For this review, take the finished solid that the model builds, in its own axes (mm). A direction names the side the tool comes from. Round coordinates to 2 decimals unless told otherwise and drop trailing zeros. Order: outer loops, then holes, each group sorted by start corner. A loop starts at its lowest first (then second) coordinate and runs counter-clockwise, first axis right, second up. Notation, with made-up numbers: (-23, 77) -> (32, 77) arc R20 cw to (32, 85) -> close; hole circle Ø6 at (48.5, 15). An arc over 180 degrees is marked (long way). Answer in a Markdown table with one row per item.
```python
from build123d import *

# Parameters (mm, degrees)
SKETCH1_R           = 1.5
BOSS_EXTRUDE1_DEPTH = 4


with BuildPart() as part:
    # Sketch1 → Boss-Extrude1 (new body)
    with BuildSketch(Plane.XY):
        with BuildLine():
            Line((3.999999567, 13.999999851), (-4.33e-07, 13.999999851))
            Line((-4.33e-07, 13.999999851), (-4.33e-07, 4.999999851))
            Line((-4.33e-07, 4.999999851), (3.999999567, 4.999999851))
            Line((3.999999567, 4.999999851), (3.999999567, -1.49e-07))
            Line((3.999999567, -1.49e-07), (51.999999567, -1.49e-07))
            Line((51.999999567, -1.49e-07), (51.999999567, 4.999999851))
            Line((51.999999567, 4.999999851), (55.999999567, 4.999999851))
            Line((55.999999567, 4.999999851), (55.999999567, 13.999999851))
            Line((55.999999567, 13.999999851), (51.999999567, 13.999999851))
            Line((51.999999567, 13.999999851), (51.999999567, 18.999999851))
            ThreePointArc((51.999999567, 18.999999851), (49.656853817, 24.6568541), (43.999999567, 26.999999851))
            Line((43.999999567, 26.999999851), (11.999999567, 26.999999851))
            ThreePointArc((11.999999567, 26.999999851), (6.343145318, 24.6568541), (3.999999567, 18.999999851))
            Line((3.999999567, 18.999999851), (3.999999567, 13.999999851))
        make_face()
        with Locations((46.999999567, 18.299999851)):
            Circle(SKETCH1_R, mode=Mode.SUBTRACT)
        with Locations((46.999999567, 8.299999851)):
            Circle(SKETCH1_R, mode=Mode.SUBTRACT)
        with Locations((18.499999567, 18.299999851)):
            Circle(SKETCH1_R, mode=Mode.SUBTRACT)
        with Locations((18.499999567, 8.299999851)):
            Circle(SKETCH1_R, mode=Mode.SUBTRACT)
    extrude(amount=BOSS_EXTRUDE1_DEPTH)


solid = part.part
```
Q1. The part is to be moulded in two halves that separate along Y. For faces 4 (the face through (4, 17, 2)), 5 (the face through (17.3, 7.4, 2)), 6 (the face through (45.8, 7.4, 2)), 7 (the face through (49.719, 24.594, 1.972)), say which applies: +Y half, -Y half, draft (parallel to the pull), parting line (faces both ways), or undercut.
Answer key:
| item | result |
|---|---|
| face 4 | draft |
| face 5 | undercut |
| face 6 | undercut |
| face 7 | +Y half |
Q2. Take a section at C-C, the plane x = 18.5. Write out the cut boundary in (y, z), then the cut area to 3 significant figures.
Answer key:
| item | result |
|---|---|
| outline | (0, 0) -> (6.8, 0) -> (6.8, 4) -> (0, 4) -> close; (9.8, 0) -> (16.8, 0) -> (16.8, 4) -> (9.8, 4) -> close; (19.8, 0) -> (27, 0) -> (27, 4) -> (19.8, 4) -> close |
| area | 84.0 mm^2 |
Q3. To check wall thickness, follow probe 1 along X at (y, z) = (8.3, 1.55); probe 2 along Y at (x, z) = (47, 2.85); probe 3 along X at (y, z) = (9.25, 3.15). State the ranges of each line that lie inside material, in increasing order.
Answer key:
| item | result |
|---|---|
| probe 1 | x = 0 to 17, 20 to 45.5, 48.5 to 56 |
| probe 2 | y = 0 to 6.8, 9.8 to 16.8, 19.8 to 26.42 |
| probe 3 | x = 0 to 17.34, 19.66 to 45.84, 48.16 to 56 |
Q4. Take a section at D-D, the plane y = 15.5. Write out the cut boundary in (x, z), then the cut area to 3 significant figures.
Answer key:
| item | result |
|---|---|
| outline | (4, 0) -> (52, 0) -> (52, 4) -> (4, 4) -> close |
| area | 192 mm^2 |
Q5. Take a section at B-B, the plane z = 2.1. Write out the cut boundary in (x, y).
Answer key:
| item | result |
|---|---|
| outline | (0, 5) -> (4, 5) -> (4, 0) -> (52, 0) -> (52, 5) -> (56, 5) -> (56, 14) -> (52, 14) -> (52, 19) arc R8 ccw to (44, 27) -> (12, 27) arc R8 ccw to (4, 19) -> (4, 14) -> (0, 14) -> close; hole circle Ø3 at (18.5, 8.3); hole circle Ø3 at (18.5, 18.3); hole circle Ø3 at (47, 8.3); hole circle Ø3 at (47, 18.3) |
Q6. Take a section at A-A, the plane y = 8.3. Write out the cut boundary in (x, z).
Answer key:
| item | result |
|---|---|
| outline | (0, 0) -> (17, 0) -> (17, 4) -> (0, 4) -> close; (20, 0) -> (45.5, 0) -> (45.5, 4) -> (20, 4) -> close; (48.5, 0) -> (56, 0) -> (56, 4) -> (48.5, 4) -> close |
Q7. Clearance check with flat-ended pins moving along their axes: pin 1 Ø1.2 at (x, z) = (3, 2.5) entering from -Y; pin 2 Ø2 at (y, z) = (15.5, 1) entering from +X; pin 3 Ø1.2 at (y, z) = (3, 3) entering from -X. State where each tip first meets the part, or that it passes through.
Answer key:
| item | result |
|---|---|
| pin 1 | stops at y = 5 |
| pin 2 | stops at x = 52 |
| pin 3 | stops at x = 4 |
Q8. Tool access review of faces 1 (the face through (52, 2, 2)), 2 (the face through (52, 16, 2)), 3 (the face through (2, 14, 2)): name each direction out of +Z, -Z, +X, -X, +Y, -Y from which nothing blocks a thin tool from reaching the whole face with its end or side.
Answer key:
| item | result |
|---|---|
| face 1 | +Z, -Z, +X, -Y |
| face 2 | +Z, -Z, +X, +Y |
| face 3 | +Z, -Z, -X, +Y |
